Model file for the job. Use its own axes, mm. Round coordinates to 2 decimals unless told otherwise and drop trailing zeros. Order: outer loops, then holes, each group sorted by start corner. A loop starts at its lowest first (then second) coordinate and runs counter-clockwise, first axis right, second up. Notation, with made-up numbers: (-39.5, 3) - (3.5, 3) arc R22 ccw to (3.5, 34) - close; hole circle Ø5 at (51, 12.5). An arc over 180 degrees is marked (long way). Put each result on its own line as item: value. Start each with the question number.
Item 1: Saw through at B-B on y = 309. List the corners of the cut face in (x, z).
Item 2: Saw through at C-C on z = 4.25. List the corners of the cut face in (x, y).
Item 3: Saw through at A-A on x = -19. List the corners of the cut face in (y, z).
Item 4: Pin check, flat tips, straight feed: pin 1 Ø17.5 at (x, y) = (-61, 351) entering from +Z; pin 2 Ø3.5 at (x, y) = (-61, 311.5) entering from +Z; pin 3 Ø5 at (x, y) = (-61, 309) entering from -Z. Stop position of each tip, or through.
Item 5: Probe probe 1 along X at (y, z) = (351, 2.9); probe 2 along X at (y, z) = (309, 10.75); probe 3 along Y at (x, z) = (-19, 4). List the from-to ranges inside material, lowest first.
Item 6: Saw through at D-D on x = 28.5. List the corners of the cut face in (y, z).
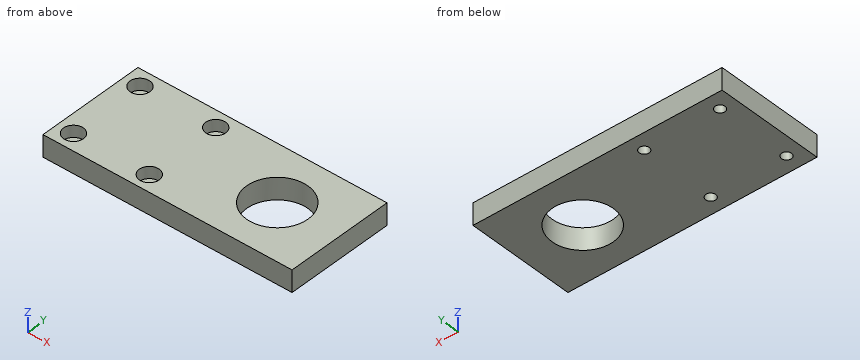
```python
from build123d import *

# Parameters (mm, degrees)
SZKIC1_W                                             = 138
SZKIC1_H                                             = 60
SZKIC1_R                                             = 17
DODANIE_WYCI_GNI_CIE1_DEPTH                          = 12
POG_BIENIE_WALCOWE_POD_M5_WKR_T_DO_CZ_CI_D           = 5.5
POG_BIENIE_WALCOWE_POD_M5_WKR_T_DO_CZ_CI_CBORE_D     = 11
POG_BIENIE_WALCOWE_POD_M5_WKR_T_DO_CZ_CI_CBORE_DEPTH = 6.5


with BuildPart() as part:
    # Szkic1 → Dodanie-wyciągnięcie1 (new body)
    with BuildSketch(Plane.XY):
        with Locations((-1, 330)):
            Rectangle(SZKIC1_W, SZKIC1_H)
        with Locations((33.5, 330)):
            Circle(SZKIC1_R, mode=Mode.SUBTRACT)
    extrude(amount=DODANIE_WYCI_GNI_CIE1_DEPTH)

    # Pogłębienie walcowe pod M5 Wkręt do części metalowych z łbem sześciokątnym1 (through all)
    with Locations(Plane.XY.offset(12)):
        with Locations((-61, 351), (-19, 351), (-61, 309), (-19, 309)):
            CounterBoreHole(POG_BIENIE_WALCOWE_POD_M5_WKR_T_DO_CZ_CI_D / 2, POG_BIENIE_WALCOWE_POD_M5_WKR_T_DO_CZ_CI_CBORE_D / 2, POG_BIENIE_WALCOWE_POD_M5_WKR_T_DO_CZ_CI_CBORE_DEPTH)


solid = part.part
```
Results found:
1. outline: (-70, 0) - (-63.75, 0) - (-63.75, 5.5) - (-66.5, 5.5) - (-66.5, 12) - (-70, 12) - close; (-58.25, 0) - (-21.75, 0) - (-21.75, 5.5) - (-24.5, 5.5) - (-24.5, 12) - (-55.5, 12) - (-55.5, 5.5) - (-58.25, 5.5) - close; (-16.25, 0) - (68, 0) - (68, 12) - (-13.5, 12) - (-13.5, 5.5) - (-16.25, 5.5) - close
2. outline: (-70, 300) - (68, 300) - (68, 360) - (-70, 360) - close; hole circle Ø5.5 at (-61, 309); hole circle Ø5.5 at (-61, 351); hole circle Ø5.5 at (-19, 309); hole circle Ø5.5 at (-19, 351); hole circle Ø34 at (33.5, 330)
3. outline: (300, 0) - (306.25, 0) - (306.25, 5.5) - (303.5, 5.5) - (303.5, 12) - (300, 12) - close; (311.75, 0) - (348.25, 0) - (348.25, 5.5) - (345.5, 5.5) - (345.5, 12) - (314.5, 12) - (314.5, 5.5) - (311.75, 5.5) - close; (353.75, 0) - (360, 0) - (360, 12) - (356.5, 12) - (356.5, 5.5) - (353.75, 5.5) - close
4. pin 1: stops at z = 12
4. pin 2: stops at z = 5.5
4. pin 3: passes through
5. probe 1: x = -70 to -63.75, -58.25 to -21.75, -16.25 to 68
5. probe 2: x = -70 to -66.5, -55.5 to -24.5, -13.5 to 68
5. probe 3: y = 300 to 306.25, 311.75 to 348.25, 353.75 to 360
6. outline: (300, 0) - (313.75, 0) - (313.75, 12) - (300, 12) - close; (346.25, 0) - (360, 0) - (360, 12) - (346.25, 12) - close
